Read the model definition and answer for the solid it produces. Units are mm, in the model's axes. A direction names the side the tool comes from. Give positions to 0.01 mm unless a question says otherwise; leave off trailing zeros. Loops run counter-clockwise (first coordinate to the right, second up) from the corner with the lowest first, then second, coordinate; pieces in that order, holes last. Notation, with made-up numbers: (73.5, 75) - (128.5, 75) arc R17 ccw to (128.5, 87) - close; hole circle Ø9 at (66, -5.5). An arc over 180 degrees is marked (long way). Write item = value, one per line.
```python
from build123d import *

# Parameters (mm, degrees)
F1_DEPTH = 100


with BuildPart() as f1:
    # F0 (on Front) → F1 (new body)
    with BuildSketch(Plane.XZ):
        with BuildLine():
            Line((1.99592, 6.5), (21.49592, 6.5))
            ThreePointArc((21.49592, 6.5), (22.203027, 6.207107), (22.49592, 5.5))
            Line((22.49592, 5.5), (22.49592, -5.5))
            ThreePointArc((22.49592, -5.5), (22.203027, -6.207107), (21.49592, -6.5))
            Line((21.49592, -6.5), (-13.00408, -6.5))
            ThreePointArc((-13.00408, -6.5), (-14.050214, -6.92501), (-14.503525, -7.959196))
            Line((-14.503525, -7.959196), (-14.504665, -8.00111))
            ThreePointArc((-14.504665, -8.00111), (-14.196328, -8.95365), (-13.357338, -9.5))
            Line((-13.357338, -9.5), (22.49592, -9.5))
            ThreePointArc((22.49592, -9.5), (24.617241, -8.62132), (25.49592, -6.5))
            Line((25.49592, -6.5), (25.49592, 5.5))
            Line((25.49592, 5.5), (25.49592, 6.5))
            ThreePointArc((25.49592, 6.5), (24.617241, 8.62132), (22.49592, 9.5))
            Line((22.49592, 9.5), (1.99592, 9.5))
            ThreePointArc((1.99592, 9.5), (0.93526, 9.06066), (0.49592, 8))
            ThreePointArc((0.49592, 8), (0.93526, 6.93934), (1.99592, 6.5))
        make_face()
    extrude(amount=F1_DEPTH)


solid = f1.part
```
1) Each of these flat-tipped pins is pushed along its axis until it touches: P1, Ø8, axis at x = -6.5, y = -61, coming from the +Z side; P2, Ø1.5, axis at y = -17.5, z = 4, coming from the -X side. Where does it stop, or does it pass through?
Output:
P1 = -6.5
P2 = 22.5
2) A cutting plane is placed at C-C on x = -10. Determine the outline of the cut face in (y, z), then the cut area to 3 significant figures.
Output:
outline = (-100, -9.5) - (0, -9.5) - (0, -6.5) - (-100, -6.5) - close
area = 300 mm²
3) A cutting plane is placed at D-D on z = -1.75. Determine the outline of the cut face in (x, y), then the cut area to 3 significant figures.
Output:
outline = (22.5, -100) - (25.5, -100) - (25.5, 0) - (22.5, 0) - close
area = 300 mm²
4) The mould has two halves that part along Z. Classify faces 3 (the face through (4, -49, -6.5)), 4 (the face through (24.64, -49.3, 8.6)), 5 (the face through (24.594, -49.3, -8.645)): pulls with the +Z half, pulls with the -Z half, needs draft (parallel to the pull), parting line crosses it, or undercut.
Output:
face_3 = undercut
face_4 = pulls with the +Z half
face_5 = pulls with the -Z half
5) A tool of negligible diameter and unlimited length cuts with its end or side. For faces 1 (the face through (12, -49, 6.5)), 2 (the face through (12, -49, 9.5)), from which of +Z, -Z, +X, -X, +Y, -Y can it reach the whole face along a straight path? Write none if from no direction.
Output:
face_1 = -X, +Y, -Y
face_2 = +Z, +X, -X, +Y, -Y
6) Find the intervals of material crossed by probe 1 along Z at (x, y) = (17.5, -91.5); probe 2 along X at (y, z) = (-8, -5.25); probe 3 along Z at (x, y) = (0, -45.5), in increasing order.
Output:
probe_1 = -9.5 to -6.5, 6.5 to 9.5
probe_2 = 22.5 to 25.5
probe_3 = -9.5 to -6.5
7) A cutting plane is placed at A-A on x = 19.5. Determine the outline of the cut face in (y, z).
Output:
outline = (-100, -9.5) - (0, -9.5) - (0, -6.5) - (-100, -6.5) - close; (-100, 6.5) - (0, 6.5) - (0, 9.5) - (-100, 9.5) - close
8) A cutting plane is placed at B-B on y = -35.5. Determine the outline of the cut face in (x, z), then the cut area to 3 significant figures.
Output:
outline = (-14.5, -8) arc R1.5 ccw to (-13.36, -9.5) - (22.5, -9.5) arc R3 ccw to (25.5, -6.5) - (25.5, 6.5) arc R3 ccw to (22.5, 9.5) - (2, 9.5) arc R1.5 ccw to (0.5, 8) arc R1.5 ccw to (2, 6.5) - (21.5, 6.5) arc R1 cw to (22.5, 5.5) - (22.5, -5.5) arc R1 cw to (21.5, -6.5) - (-13, -6.5) arc R1.5 ccw to (-14.5, -7.96) - close
area = 229 mm²
